The model under review builds one solid part; all positions refer to its coordinate system, in mm. Give positions to 0.01 mm unless a question says otherwise; leave off trailing zeros. Write each loop counter-clockwise with the first axis right and the second up, starting at its lowest first coordinate (ties: lowest second). Pieces come first, ordered by that corner, then holes. Notation, with made-up numbers: M -8,10 L 12,10 A26 cw 12,35 Z; hole C 53.5,56.5 d4. An arc over 180 degrees is marked long. Write item = value, one per line. Start each with the question number.
```python
from build123d import *

# Parameters (mm, degrees)
SKETCH1_W           = 90
SKETCH1_H           = 35
SKETCH1_W_2         = 3
SKETCH1_H_2         = 15
BOSS_EXTRUDE1_DEPTH = 1.5


with BuildPart() as part:
    # Sketch1 → Boss-Extrude1 (new, symmetric)
    with BuildSketch(Plane.XY):
        Rectangle(SKETCH1_W, SKETCH1_H)
        with Locations((-46.5, 0)):
            Rectangle(SKETCH1_W_2, SKETCH1_H_2)
    extrude(amount=BOSS_EXTRUDE1_DEPTH, both=True)


solid = part.part
```
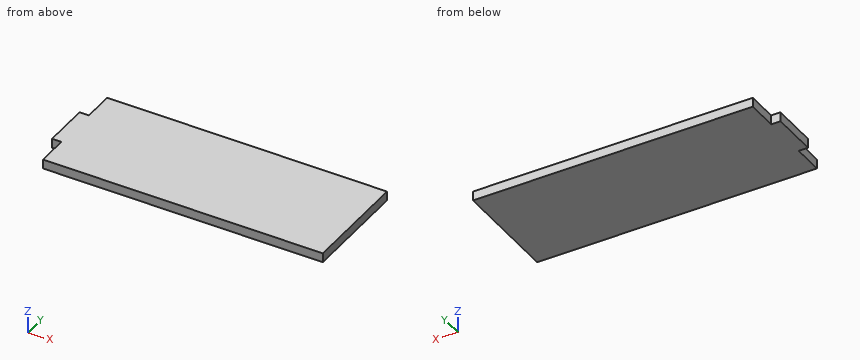
Item 1: Clearance check with flat-ended pins moving along their axes: P1, Ø1.5, axis at y = 10.5, z = 0, coming from the -X side; P2, Ø1.5, axis at x = -46.5, z = -0.5, coming from the -Y side. State where each tip first meets the part, or that it passes through.
Item 2: We need section B-B, the plane y = -10. Write out the cut boundary in (x, z).
Item 3: We need section A-A, the plane z = -0.4. Write out the cut boundary in (x, y), and give its area (4 significant figures).
Item 4: To check wall thickness, follow probe 1 along X at (y, z) = (11, -0.5). State the ranges of the line that lie inside material, in increasing order. Write a range as [from, to].
Worked out:
q1.P1 = -45
q1.P2 = -7.5
q2.outline = M -45,-1.5 L 45,-1.5 L 45,1.5 L -45,1.5 Z
q3.outline = M -48,-7.5 L -45,-7.5 L -45,-17.5 L 45,-17.5 L 45,17.5 L -45,17.5 L -45,7.5 L -48,7.5 Z
q3.area = 3,195 mm²
q4.probe_1 = [-45, 45]
